```python
from build123d import *

# Parameters (mm, degrees)
CYLINDER082_R           = 1.7
CYLINDER082_DEPTH       = 50
CYLINDER081_R           = 1.7
CYLINDER081_DEPTH       = 50
CYLINDER080_R           = 1.7
CYLINDER080_DEPTH       = 50
CYLINDER079_R           = 1.7
CYLINDER079_DEPTH       = 50
CYLINDER044_R           = 3.5
CYLINDER044_DEPTH       = 8
CYLINDER044_PITCH_ANGLE = 90
BOX027_W                = 2
BOX027_H                = 7
BOX027_DEPTH            = 10
BOX019_W                = 66
BOX019_H                = 50
BOX019_DEPTH            = 25
BOX019_PLACEMENT_ANGLE  = -7
BOX010_W                = 10
BOX010_H                = 40
BOX010_DEPTH            = 4
CYLINDER024_R           = 6
CYLINDER024_DEPTH       = 4


with BuildPart() as m3_studding019:
    # Cylinder082 → Cylinder082 (new body)
    with BuildSketch(Plane(origin=(41, -9, 27), x_dir=(1, 0, 0), z_dir=(0, 0, 1))):
        Circle(CYLINDER082_R)
    extrude(amount=CYLINDER082_DEPTH)


with BuildPart() as m3_studding018:
    # Cylinder081 → Cylinder081 (new body)
    with BuildSketch(Plane(origin=(42, 22, 27), x_dir=(1, 0, 0), z_dir=(0, 0, 1))):
        Circle(CYLINDER081_R)
    extrude(amount=CYLINDER081_DEPTH)


with BuildPart() as m3_studding017:
    # Cylinder080 → Cylinder080 (new body)
    with BuildSketch(Plane(origin=(42.5, 7, 27), x_dir=(1, 0, 0), z_dir=(0, 0, 1))):
        Circle(CYLINDER080_R)
    extrude(amount=CYLINDER080_DEPTH)


with BuildPart() as m3_clearance003:
    # Cylinder079 → Cylinder079 (new body)
    with BuildSketch(Plane(origin=(36, 0, 27), x_dir=(1, 0, 0), z_dir=(0, 0, 1))):
        Circle(CYLINDER079_R)
    extrude(amount=CYLINDER079_DEPTH)

    # Fusion048: union m3-studding019, m3-studding018, m3-studding017
    add(m3_studding019.part)
    add(m3_studding018.part)
    add(m3_studding017.part)


with BuildPart() as cylinder044:
    # Cylinder044 → Cylinder044 (new body)
    with BuildSketch(Plane.XY):
        Circle(CYLINDER044_R)
    extrude(amount=CYLINDER044_DEPTH)


with BuildPart() as cylinder044_1:
    # Cylinder044 pitch: moved
    add(cylinder044.part.rotate(Axis((0, 0, 0), (0, 1, 0)), CYLINDER044_PITCH_ANGLE))


with BuildPart() as cylinder044_2:
    # Cylinder044 placement: moved
    add(cylinder044_1.part.moved(Location((41, 15, 58))))


with BuildPart() as obj1:
    # Box027 → Box027 (new body)
    with BuildSketch(Plane(origin=(41, 11.5, 58), x_dir=(1, 0, 0), z_dir=(0, 0, 1))):
        with Locations((1, 3.5)):
            Rectangle(BOX027_W, BOX027_H)
    extrude(amount=BOX027_DEPTH)

    # Fusion026: union Cylinder044
    add(cylinder044_2.part)


with BuildPart() as cube019:
    # Box019 → Box019 (new body)
    with BuildSketch(Plane.XY):
        with Locations((33, 25)):
            Rectangle(BOX019_W, BOX019_H)
    extrude(amount=BOX019_DEPTH)


with BuildPart() as cube019_1:
    # Box019 placement: moved
    add(cube019.part.moved(Location((-31.823564, -10.815, 45))).rotate(Axis((-31.823564, -10.815, 45), (0, 0, 1)), BOX019_PLACEMENT_ANGLE))


with BuildPart() as cut008:
    # Box010 → Box010 (new body)
    with BuildSketch(Plane(origin=(36, -15, 60.7), x_dir=(1, 0, 0), z_dir=(0, 0, 1))):
        with Locations((5, 20)):
            Rectangle(BOX010_W, BOX010_H)
    extrude(amount=BOX010_DEPTH)

    # Cut008: cut Cube019
    add(cube019_1.part, mode=Mode.SUBTRACT)


with BuildPart() as clamp_plate:
    # Cylinder024 → Cylinder024 (new body)
    with BuildSketch(Plane(origin=(38, 0, 60.7), x_dir=(1, 0, 0), z_dir=(0, 0, 1))):
        Circle(CYLINDER024_R)
    extrude(amount=CYLINDER024_DEPTH)

    # Fusion013: union Cut008
    add(cut008.part)

    # Cut016: cut obj1
    add(obj1.part, mode=Mode.SUBTRACT)

    # Cut038: cut M3-clearance003
    add(m3_clearance003.part, mode=Mode.SUBTRACT)


with BuildPart() as clamp_plate_1:
    # Cut038 placement: moved
    add(clamp_plate.part.moved(Location((-0.5, 0, 0))))


solid = clamp_plate_1.part
```
The model under review builds one solid part; all positions refer to its coordinate system, in mm. A direction names the side the tool comes from. Give positions to 0.01 mm unless a question says otherwise; leave off trailing zeros. Loops run counter-clockwise (first coordinate to the right, second up) from the corner with the lowest first, then second, coordinate; pieces in that order, holes last. Notation, with made-up numbers: (-16.75, 80) -> (1.25, 80) arc R24 ccw to (1.25, 97) -> close; hole circle Ø10 at (87, -9). An arc over 180 degrees is marked (long way). Use CSV: the item, a comma, the result in double quotes.
1. Consider section A-A, the plane y = 0. Write out the cut boundary in (x, z), then the cut area to 3 significant figures.
Result:
outline,"(31.5, 60.7) -> (33.8, 60.7) -> (33.8, 64.7) -> (31.5, 64.7) -> close; (37.2, 60.7) -> (45.5, 60.7) -> (45.5, 64.7) -> (37.2, 64.7) -> close"
area,"42.4 mm²"
2. Machinability: for faces 4 (the face through (42, 25, 63)), 5 (the face through (44, 15, 61.5)), 6 (the face through (40.5, 15, 63)), 7 (the face through (35.5, -10, 63)), which of the approach directions +Z, -Z, +X, -X, +Y, -Y give a long, thin tool a straight path to every point of the face, cutting with its end or side? Answer none if there is none.
Result:
face 4,"+Z, -Z, +X, -X, +Y"
face 5,"-Z, +X"
face 6,"+Z, -Z"
face 7,"+Z, -Z, -X, -Y"
3. To check wall thickness, follow probe 1 along Y at (x, z) = (41.5, 61.7); probe 2 along X at (y, z) = (-9, 62.1); probe 3 along X at (y, z) = (0, 62). State the ranges of each line that lie inside material, in increasing order. Write a range as from..to.
Result:
probe 1,"y = -15..-10.37, -7.63..5.38, 8.62..11.5, 18.5..20.3, 23.7..25"
probe 2,"x = 35.5..38.8, 42.2..45.5"
probe 3,"x = 31.5..33.8, 37.2..45.5"
4. For P1, Ø2.5, axis at x = 42, y = 7, coming from the -Z side; P2, Ø1, axis at x = 34, z = 62, coming from the -Y side, all flat-tipped, find the tip position at first contact; note any pin that passes through.
Result:
P1,"passes through"
P2,"stops at y = -5.2"
5. Consider section C-C, the plane x = 41. Write out the cut boundary in (y, z).
Result:
outline,"(-15, 60.7) -> (-10.62, 60.7) -> (-10.62, 64.7) -> (-15, 64.7) -> close; (-7.38, 60.7) -> (5.63, 60.7) -> (5.63, 64.7) -> (-7.38, 64.7) -> close; (8.37, 60.7) -> (11.5, 60.7) -> (11.5, 64.7) -> (8.37, 64.7) -> close; (18.5, 60.7) -> (20.38, 60.7) -> (20.38, 64.7) -> (18.5, 64.7) -> close; (23.62, 60.7) -> (25, 60.7) -> (25, 64.7) -> (23.62, 64.7) -> close"
6. Consider section D-D, the plane x = 34.25. Write out the cut boundary in (y, z), then the cut area to 3 significant figures.
Result:
outline,"(-5.04, 60.7) -> (-1.15, 60.7) -> (-1.15, 64.7) -> (-5.04, 64.7) -> close; (1.15, 60.7) -> (5.04, 60.7) -> (5.04, 64.7) -> (1.15, 64.7) -> close"
area,"31.1 mm²"
7. The part is to be moulded in two halves that separate along X. For faces 1 (the face through (45.5, 5, 63)), 2 (the face through (42.5, 15, 63)), 3 (the face through (40, 5, 60.7)), say which applies: +X half, -X half, draft (parallel to the pull), parting line (faces both ways), or undercut.
Result:
face 1,"+X half"
face 2,"undercut"
face 3,"draft"
8. Consider section B-B, the plane z = 63.45. Write out the cut boundary in (x, y), then the cut area to 3 significant figures.
Result:
outline,"(35.5, -15) -> (45.5, -15) -> (45.5, 25) -> (38.57, 25) -> (36.22, 5.86) arc R6 ccw to (35.5, -5.66) -> close; hole circle Ø3.4 at (35.5, 0); hole circle Ø3.4 at (40.5, -9); hole circle Ø3.4 at (41.5, 22); hole circle Ø3.4 at (42, 7); hole (40.5, 11.5) -> (42.5, 11.5) -> (42.5, 18.5) -> (40.5, 18.5) -> close"
area,"346 mm²"
